Geometry: final body of the model. Coordinates: model frame, mm. A direction names the side the tool comes from. Give positions to 0.01 mm unless a question says otherwise; leave off trailing zeros. Write each loop counter-clockwise with the first axis right and the second up, starting at its lowest first coordinate (ties: lowest second). Pieces come first, ordered by that corner, then holes.
Q1. Mould query, pull axis X, two halves, no side actions, for faces 1 (the flat face through (25, 8, 11.5)), 2 (the flat face through (27, 8, 10.805)), 3 (the flat face through (1.55, 14.93, 1.21)), 4 (the flat face through (28.5, 8.2, 38)). Classes: +X half, -X half, draft (parallel to the pull), parting line (faces both ways), or undercut.
Q2. Pin query (flat end, axial travel): pin 1 Ø4 at (x, y) = (11, 7) entering from +Z; pin 2 Ø3.5 at (x, y) = (25, 7.5) entering from +Z; pin 3 Ø5 at (x, y) = (3, 5.5) entering from +Z; pin 4 Ø1.6 at (y, z) = (1, 7.5) entering from -X. Return the tip coordinate at first contact, or that it passes through.
Q3. Section D-D (z = 34.5). Return the cut outline in (x, y).
Q4. Reachability of faces 5 (the flat face through (27, 8, 21)), 6 (the flat face through (6.464, 1, 7)), 7 (the flat face through (23.536, 15, 7)) from +Z, -Z, +X, -X, +Y, -Y: full face, straight path, thin tool, end or side. Return the list, or none.
Q5. Section A-A (y = 8.25). Return the cut outline in (x, z) (3 decimals).
Q6. Section B-B (x = 4.75). Return the cut outline in (y, z), plus the area to 3 significant figures.
Q7. Section C-C (z = 3.5). Return the cut outline in (x, y), plus the area to 4 significant figures.
Q8. Line query: line 1 (X direction, y = 10, z = 35.5); line 2 (Z direction, x = 23.95, y = 8.25); line 3 (Y direction, x = 22.5, z = 36). Output: solid intervals per line, ascending.
from build123d import *

# Parameters (mm, degrees)
F0_W      = 29
F0_H      = 16.5
F1_DEPTH  = 38.5
F2_T      = -2
F3_DEPTH  = 2.25
F4_SIZE   = 2
F5_SIZE   = 2
F6_SIZE   = 1
F8_DEPTH  = 16.501
F9_W      = 7.54
F9_H      = 7.25
F9_R      = 1.1
F10_DEPTH = 6.35
F13_W     = 5.538
F13_H     = 4.583
F11_W     = 5.538
F11_H     = 5.533


with BuildPart() as f1:
    # F0 (on Top) → F1 (new body)
    with BuildSketch(Plane.XY):
        with Locations((14.5, 8.25)):
            Rectangle(F0_W, F0_H)
    extrude(amount=F1_DEPTH)

    # F2
    f2_openings = [f1.faces().sort_by_distance(p)[0] for p in [
        (14.5, 8.25, 38.5),
    ]]
    offset(amount=F2_T, openings=f2_openings)

    # F3 (add): a face of the model
    f3_faces = [f1.faces().sort_by_distance(p)[0] for p in [
        (14.5, 8.25, 2),
    ]]
    extrude(f3_faces, amount=F3_DEPTH)

    # F4
    f4_edges = [f1.edges().sort_by_distance(p)[0] for p in [
        (29, 0, 19.25),
        (29, 16.5, 19.25),
        (0, 16.5, 19.25),
        (0, 0, 19.25),
    ]]
    chamfer(f4_edges, length=F4_SIZE)

    # F5
    f5_edges = [f1.edges().sort_by_distance(p)[0] for p in [
        (0, 8.25, 0),
        (1, 15.5, 0),
        (1, 1, 0),
        (14.5, 16.5, 0),
        (14.5, 0, 0),
        (28, 15.5, 0),
        (28, 1, 0),
        (29, 8.25, 0),
    ]]
    chamfer(f5_edges, length=F5_SIZE)

    # F6
    f6_edges = [f1.edges().sort_by_distance(p)[0] for p in [
        (0, 8.25, 38.5),
        (1, 1, 38.5),
        (14.5, 0, 38.5),
        (28, 1, 38.5),
        (29, 8.25, 38.5),
        (28, 15.5, 38.5),
        (14.5, 16.5, 38.5),
        (1, 15.5, 38.5),
    ]]
    chamfer(f6_edges, length=F6_SIZE)

    # F7 (on face) → F8 (cut, through all)
    with BuildSketch(Plane.XZ):
        Polygon((23.536, 8.664), (17.365, 12.824), (12.635, 12.824), (6.464, 8.664), (6.464, 4.94), (23.536, 4.94), align=None)
    extrude(amount=-F8_DEPTH, mode=Mode.SUBTRACT)

    # F9 (on face) → F10 (join)
    with BuildSketch(Plane.YZ.offset(29)):
        with Locations((8.25, 7.875)):
            Rectangle(F9_W, F9_H)
        with Locations((8.25, 9)):
            Circle(F9_R, mode=Mode.SUBTRACT)
    extrude(amount=-F10_DEPTH)

    # F13 (on offset) → F14 section 0
    with BuildSketch(Plane.YZ.offset(24.55)):
        with Locations((8.25, 8.5135)):
            Rectangle(F13_W, F13_H)
    # F11 (on face) → F14 section 1
    with BuildSketch(Plane.YZ.offset(29)):
        with Locations((8.25, 8.0385)):
            Rectangle(F11_W, F11_H)
    loft(mode=Mode.SUBTRACT)


solid = f1.part
Computed:
1. face 1: undercut
1. face 2: draft
1. face 3: -X half
1. face 4: +X half
2. pin 1: stops at z = 4.25
2. pin 2: stops at z = 11.5
2. pin 3: stops at z = 38.5
2. pin 4: stops at x = 0.2
3. outline: (0, 2) - (2, 0) - (27, 0) - (29, 2) - (29, 14.5) - (27, 16.5) - (2, 16.5) - (0, 14.5) - close; hole (2, 2) - (27, 2) - (27, 14.5) - (2, 14.5) - close
4. face 5: +Z
4. face 6: +Y, -Y
4. face 7: +Y
5. outline: (0, 2) - (2, 0) - (27, 0) - (29, 2) - (29, 5.272) - (24.55, 6.222) - (24.55, 7.9) - (22.65, 7.9) - (22.65, 4.25) - (2, 4.25) - (2, 38.5) - (1, 38.5) - (0, 37.5) - close; (22.65, 10.1) - (24.55, 10.1) - (24.55, 10.805) - (29, 10.805) - (29, 37.5) - (28, 38.5) - (27, 38.5) - (27, 11.5) - (22.65, 11.5) - close
6. outline: (0, 2) - (2, 0) - (14.5, 0) - (16.5, 2) - (16.5, 37.5) - (15.5, 38.5) - (14.5, 38.5) - (14.5, 4.25) - (2, 4.25) - (2, 38.5) - (1, 38.5) - (0, 37.5) - close
6. area: 202 mm2
7. outline: (0, 2) - (2, 0) - (27, 0) - (29, 2) - (29, 14.5) - (27, 16.5) - (2, 16.5) - (0, 14.5) - close
7. area: 470.5 mm2
8. line 1: x = 0 to 2, 27 to 29
8. line 2: z = 0 to 7.9, 10.1 to 11.5
8. line 3: y = 0 to 2, 14.5 to 16.5
